Build history of the part. All positions in model axes, mm. Coordinates: 2 decimals unless noted, no trailing zeros. Order: outer loops, then holes, each group sorted by start corner. A loop starts at its lowest first (then second) coordinate and runs counter-clockwise, first axis right, second up. Notation, with made-up numbers: M -13.5,-10.75 L 32.5,-10.75 A29 cw 32.5,16.25 Z; hole C 43,87.5 d10. An arc over 180 degrees is marked long. Use a Markdown table: item, result. Add a question column.
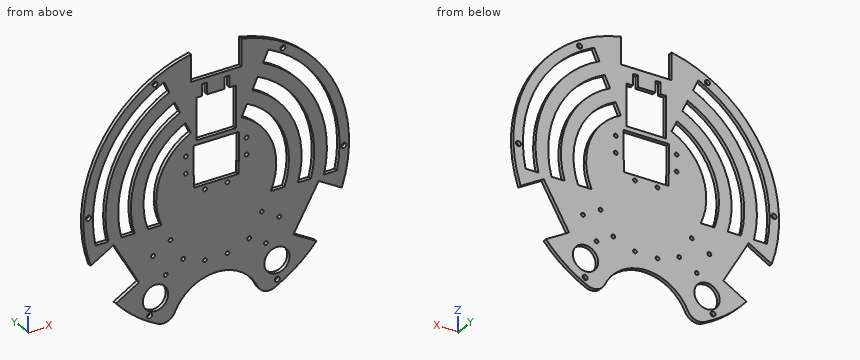
from build123d import *

# Parameters (mm, degrees)
CROQUIS1_R              = 105
SALIENTE_EXTRUIR1_DEPTH = 3
CORTAR_EXTRUIR1_START   = -3
CORTAR_EXTRUIR1_DEPTH   = 3
REDONDEO1_R             = 10
CROQUIS3_W              = 40
CROQUIS3_H              = 28
CORTAR_EXTRUIR12_DEPTH  = 149.522725677
CROQUIS12_W             = 31
CROQUIS12_H             = 32.5
CROQUIS12_W_2           = 36
CROQUIS12_H_2           = 23
CORTAR_EXTRUIR13_DEPTH  = 148.169969906
CROQUIS15_R             = 1.5
CROQUIS15_W             = 35
CROQUIS15_H             = 9
CORTAR_EXTRUIR17_DEPTH  = 148.169969906
CROQUIS16_R             = 10
CROQUIS16_R_2           = 2
CORTAR_EXTRUIR18_DEPTH  = 10
CROQUIS18_R             = 1.5
CORTAR_EXTRUIR19_DEPTH  = 148.169969906
CROQUIS19_W             = 4
CROQUIS19_H             = 9
CORTAR_EXTRUIR20_DEPTH  = 148.169969906


with BuildPart() as part:
    # Croquis1 → Saliente-Extruir1 (new body)
    with BuildSketch(Plane(origin=(0, 0, 0), x_dir=(1, 0, 0), z_dir=(0, 1, 0))):
        with Locations(Location((0, 0, 0), (0, 0, 270))):
            Circle(CROQUIS1_R)
    extrude(amount=SALIENTE_EXTRUIR1_DEPTH)

    # Croquis2 → Cortar-Extruir1 (cut)
    with BuildSketch(Plane(origin=(0, 3, 0), x_dir=(1, 0, 0), z_dir=(0, 1, 0)).offset(CORTAR_EXTRUIR1_START)):
        with BuildLine():
            ThreePointArc((35.71668902, 98.738635424), (0, 68.738635424), (-35.71668902, 98.738635424))
            ThreePointArc((-35.71668902, 98.738635424), (0, 105), (35.71668902, 98.738635424))
        make_face()
    extrude(amount=CORTAR_EXTRUIR1_DEPTH, mode=Mode.SUBTRACT)

    # Redondeo1
    redondeo1_edges = [part.edges().sort_by_distance(p)[0] for p in [
        (-35.71668902, 1.5, -98.738635424),
        (35.71668902, 1.5, -98.738635424),
    ]]
    fillet(redondeo1_edges, radius=REDONDEO1_R)

    # Croquis3 → Cortar-Extruir12 (cut, through all)
    with BuildSketch(Plane(origin=(0, 3, 0), x_dir=(1, 0, 0), z_dir=(0, 1, 0))):
        Polygon((-61.01408311, 58.320508076), (-85.262794416, 72.320508076), (-105.262794416, 37.679491924), (-81.01408311, 23.679491924), align=None)
        with Locations((0, -96)):
            Rectangle(CROQUIS3_W, CROQUIS3_H)
        Polygon((81.01408311, 23.679491924), (105.262794416, 37.679491924), (85.262794416, 72.320508076), (61.01408311, 58.320508076), align=None)
    extrude(amount=-CORTAR_EXTRUIR12_DEPTH, mode=Mode.SUBTRACT)

    # Croquis12 → Cortar-Extruir13 (cut, through all)
    with BuildSketch(Plane(origin=(0, 3, 0), x_dir=(1, 0, 0), z_dir=(0, 1, 0))):
        with Locations((0, -52.516645147)):
            Rectangle(CROQUIS12_W, CROQUIS12_H)
        with Locations((0, -21.266645147)):
            Rectangle(CROQUIS12_W_2, CROQUIS12_H_2)
    extrude(amount=-CORTAR_EXTRUIR13_DEPTH, mode=Mode.SUBTRACT)

    # Croquis15 → Cortar-Extruir17 (cut, through all)
    with BuildSketch(Plane(origin=(0, 3, 0), x_dir=(1, 0, 0), z_dir=(0, 1, 0))):
        with Locations(Location((-24, -13.496645147, 0), (0, 0, 270))):
            Circle(CROQUIS15_R)
        with Locations(Location((-24, -26.496645147, 0), (0, 0, 270))):
            Circle(CROQUIS15_R)
        with Locations(Location((24, -26.496645147, 0), (0, 0, 90))):
            Circle(CROQUIS15_R)
        with Locations(Location((24, -13.496645147, 0), (0, 0, 90))):
            Circle(CROQUIS15_R)
        with Locations(Location((-8.9, 57, 0), (0, 0, 270))):
            Circle(CROQUIS15_R)
        with Locations(Location((-8.9, 3, 0), (0, 0, 270))):
            Circle(CROQUIS15_R)
        with Locations(Location((8.9, 3, 0), (0, 0, 90))):
            Circle(CROQUIS15_R)
        with Locations(Location((8.9, 57, 0), (0, 0, 90))):
            Circle(CROQUIS15_R)
        with Locations((0, -5.266645147)):
            Rectangle(CROQUIS15_W, CROQUIS15_H)
    extrude(amount=-CORTAR_EXTRUIR17_DEPTH, mode=Mode.SUBTRACT)

    # Croquis16 → Cortar-Extruir18 (cut)
    with BuildSketch(Plane(origin=(0, 3, 0), x_dir=(1, 0, 0), z_dir=(0, 1, 0))):
        with Locations(Location((-48, 74, 0), (0, 0, 270))):
            Circle(CROQUIS16_R)
        with Locations(Location((48, 74, 0), (0, 0, 270))):
            Circle(CROQUIS16_R)
        with Locations(Location((-100.96794432, -2.544448812, 0), (0, 0, 270))):
            Circle(CROQUIS16_R_2)
        with Locations(Location((-52.68752947, 86.168580343, 0), (0, 0, 270))):
            Circle(CROQUIS16_R_2)
        with Locations(Location((48.28041485, 88.713029155, 0), (0, 0, 270))):
            Circle(CROQUIS16_R_2)
        with Locations(Location((100.96794432, 2.544448812, 0), (0, 0, 270))):
            Circle(CROQUIS16_R_2)
        with Locations(Location((52.68752947, -86.168580343, 0), (0, 0, 270))):
            Circle(CROQUIS16_R_2)
        with Locations(Location((-48.28041485, -88.713029155, 0), (0, 0, 270))):
            Circle(CROQUIS16_R_2)
        with BuildLine():
            Line((36.979097902, -79.301931366), (41.20528052, -88.365009236))
            ThreePointArc((41.20528052, -88.365009236), (87.194131202, -43.628356421), (95.42667342, 20))
            Line((95.42667342, 20), (85.183625187, 20))
            ThreePointArc((85.183625187, 20), (78.715634542, -38.211240213), (36.979097902, -79.301931366))
        make_face()
        with BuildLine():
            Line((64.468984791, 20), (74.874895659, 20))
            ThreePointArc((74.874895659, 20), (70.226057074, -32.780343314), (32.752915285, -70.238853495))
            Line((32.752915285, -70.238853495), (28.526732667, -61.175775625))
            ThreePointArc((28.526732667, -61.175775625), (61.720559812, -27.328053288), (64.468984791, 20))
        make_face()
        with BuildLine():
            Line((24.30055005, -52.112697755), (20.074367433, -43.049619884))
            ThreePointArc((20.074367433, -43.049619884), (44.621356196, -16.28448867), (43.084219849, 20))
            Line((43.084219849, 20), (53.909646632, 20))
            ThreePointArc((53.909646632, 20), (53.190873377, -21.839894445), (24.30055005, -52.112697755))
        make_face()
        with BuildLine():
            Line((-20.074367433, -43.049619884), (-24.30055005, -52.112697755))
            ThreePointArc((-24.30055005, -52.112697755), (-53.190873377, -21.839894445), (-53.909646632, 20))
            Line((-53.909646632, 20), (-43.084219849, 20))
            ThreePointArc((-43.084219849, 20), (-44.621356196, -16.28448867), (-20.074367433, -43.049619884))
        make_face()
        with BuildLine():
            Line((-28.526732667, -61.175775625), (-32.752915285, -70.238853495))
            ThreePointArc((-32.752915285, -70.238853495), (-70.226057074, -32.780343314), (-74.874895659, 20))
            Line((-74.874895659, 20), (-64.468984791, 20))
            ThreePointArc((-64.468984791, 20), (-61.720559812, -27.328053288), (-28.526732667, -61.175775625))
        make_face()
        with BuildLine():
            Line((-36.979097902, -79.301931366), (-41.20528052, -88.365009236))
            ThreePointArc((-41.20528052, -88.365009236), (-87.194131202, -43.628356421), (-95.42667342, 20))
            Line((-95.42667342, 20), (-85.183625187, 20))
            ThreePointArc((-85.183625187, 20), (-78.715634542, -38.211240213), (-36.979097902, -79.301931366))
        make_face()
    extrude(amount=-CORTAR_EXTRUIR18_DEPTH, mode=Mode.SUBTRACT)

    # Croquis18 → Cortar-Extruir19 (cut, through all)
    with BuildSketch(Plane(origin=(0, 3, 0), x_dir=(1, 0, 0), z_dir=(0, 1, 0))):
        with Locations(Location((-26.063193163, 50.851713533, 0), (0, 0, 270))):
            Circle(CROQUIS18_R)
        with Locations(Location((-39.924386076, 58.843417422, 0), (0, 0, 270))):
            Circle(CROQUIS18_R)
        with Locations(Location((-36.072108797, 33.524806485, 0), (0, 0, 270))):
            Circle(CROQUIS18_R)
        with Locations(Location((-49.933301709, 41.516510374, 0), (0, 0, 270))):
            Circle(CROQUIS18_R)
        with Locations(Location((36.072108797, 33.524806485, 0), (0, 0, 90))):
            Circle(CROQUIS18_R)
        with Locations(Location((49.933301709, 41.516510374, 0), (0, 0, 90))):
            Circle(CROQUIS18_R)
        with Locations(Location((26.063193163, 50.851713533, 0), (0, 0, 90))):
            Circle(CROQUIS18_R)
        with Locations(Location((39.27408311, 58.473890173, 0), (0, 0, 90))):
            Circle(CROQUIS18_R)
    extrude(amount=-CORTAR_EXTRUIR19_DEPTH, mode=Mode.SUBTRACT)

    # Croquis19 → Cortar-Extruir20 (cut, through all)
    with BuildSketch(Plane(origin=(0, 3, 0), x_dir=(1, 0, 0), z_dir=(0, 1, 0))):
        with Locations((-9.2, -73.266645147)):
            Rectangle(CROQUIS19_W, CROQUIS19_H)
        with Locations((8.5, -73.266645147)):
            Rectangle(CROQUIS19_W, CROQUIS19_H)
    extrude(amount=-CORTAR_EXTRUIR20_DEPTH, mode=Mode.SUBTRACT)


solid = part.part
(1) Slice it at C-C on y = 2.5. State how many separate pieces and enclosed holes the cut face has, and give its area (3 significant figures).
(2) Drop flat-ended pins along their axis: P1, Ø0.6, axis at x = 17.5, y = 1, coming from the +Z side; P2, Ø1.5, axis at x = -46.5, y = 1, coming from the +Z side; P3, Ø1.5, axis at x = 47.5, y = 1, coming from the +Z side; P4, Ø3.5, axis at x = 39.27, z = -58.47, coming from the +Y side. Give the stop position or say it passes through.
(3) Drill centre lines: line 1 along Z through (x, y) = (-25, 2.45); line 2 along Z through (x, y) = (-12, 0.9); line 3 along Z through (x, y) = (24, 1.45). Where is each one in solid material? Low to high. Write a range as from..to.
(4) Slice it at B-B on z = -74. Give the cut face in (x, y), and give its area (3 significant figures).
(5) Slice it at A-A on x = 91.5. Give the cut face in (y, z), and give its area (3 significant figures).
Solutions:
| question | item | result |
|---|---|---|
| 1 | separate pieces | 1 |
| 1 | enclosed holes | 32 |
| 1 | area | 20,800 mm² |
| 2 | P1 | z = 82 |
| 2 | P2 | z = 94.51 |
| 2 | P3 | z = 94.02 |
| 2 | P4 | y = 3 |
| 3 | line 1 | -78.73..-51.91, -49.79..12.38, 14.61..25.38, 27.61..40.39, 51.78..101.98 |
| 3 | line 2 | -70.78..0.77, 32.77..36.27, 68.77..82 |
| 3 | line 3 | -77.82..12, 15..25, 28..40.99, 51.47..102.22 |
| 4 | outline | M -74.49,0 L -58,0 L -58,3 L -74.49,3 Z; M -38,0 L -18.81,0 L -18.81,3 L -38,3 Z; M 18.81,0 L 38,0 L 38,3 L 18.81,3 Z; M 58,0 L 74.49,0 L 74.49,3 L 58,3 Z |
| 4 | area | 214 mm² |
| 5 | outline | M 0,-29.73 L 3,-29.73 L 3,-20 L 0,-20 Z; M 0,33.67 L 3,33.67 L 3,51.5 L 0,51.5 Z |
| 5 | area | 82.7 mm² |
